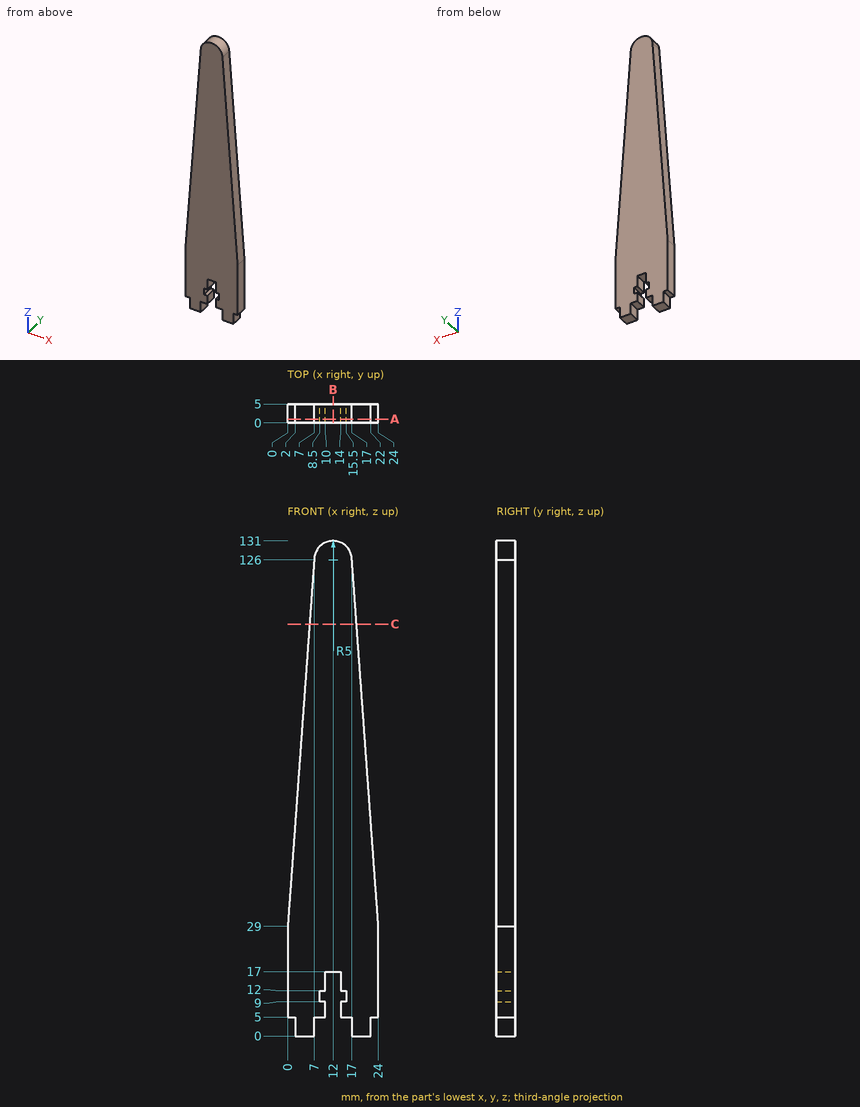
The drawing under review shows one solid part. Ordinate dimensions are in mm from its lowest x, y, z. Round coordinates to 2 decimals unless told otherwise and drop trailing zeros. Write each loop counter-clockwise with the first axis right and the second up, starting at its lowest first coordinate (ties: lowest second). Pieces come first, ordered by that corner, then holes.
(1) We need section A-A on y = 1. Give the boundary of the cut face in (x, z), and give its area (3 significant figures).
(2) We need section C-C on z = 109. Give the boundary of the cut face in (x, y), and give its area (3 significant figures).
(3) Wall thickness on L1, parallel to Z at x = 11.5, y = 3.4; L2, parallel to X at y = 1.8, z = 93.5; L3, parallel to Z at x = 9, y = 2.2: over which ranges is each line inside the solid? List them lowest first.
(4) Insertion check: pin 1 (1.2 mm diameter, centred on x = 9, y = 3, fed in from +Z); pin 2 (1 mm diameter, centred on x = 0.5, y = 2, fed in from -Z); pin 3 (1.5 mm diameter, centred on x = 9.5, y = 1.5, fed in from +Z); pin 4 (1 mm diameter, centred on x = 3.5, z = 108.5, fed in from +Y). Each pin has a flat end and moves straight along its axis. Give the tip position at first contact, or say it passes through.
(5) We need section B-B on x = 12. Give the boundary of the cut face in (y, z), and give its area (3 significant figures).
Findings below:
1. outline: (0, 5) - (2, 5) - (2, 0) - (7, 0) - (7, 5) - (10, 5) - (10, 9) - (8.5, 9) - (8.5, 12) - (10, 12) - (10, 17) - (14, 17) - (14, 12) - (15.5, 12) - (15.5, 9) - (14, 9) - (14, 5) - (17, 5) - (17, 0) - (22, 0) - (22, 5) - (24, 5) - (24, 29) - (17, 126) arc R5 ccw to (7, 126) - (0, 29) - close
1. area: 2,260 mm2
2. outline: (5.77, 0) - (18.23, 0) - (18.23, 5) - (5.77, 5) - close
2. area: 62.3 mm2
3. L1: z = 17 to 130.97
3. L2: x = 4.65 to 19.35
3. L3: z = 5 to 9, 12 to 130
4. pin 1: stops at z = 130.39
4. pin 2: stops at z = 5
4. pin 3: stops at z = 130.68
4. pin 4: passes through
5. outline: (0, 17) - (5, 17) - (5, 131) - (0, 131) - close
5. area: 570 mm2
